```python
from build123d import *

# Parameters (mm, degrees)
SKETCH5_W           = 90
SKETCH5_H           = 80
BOSS_EXTRUDE4_DEPTH = 13
BOSS_EXTRUDE5_DEPTH = 80
CHAMFER1_SIZE       = 7
SKETCH13_R          = 2
CUT_EXTRUDE4_DEPTH  = 20
SKETCH14_R          = 2
CUT_EXTRUDE8_DEPTH  = 20


with BuildPart() as part:
    # Sketch5 → Boss-Extrude4 (new body)
    with BuildSketch(Plane.XY):
        with Locations((0, -5.742449829)):
            Rectangle(SKETCH5_W, SKETCH5_H)
    extrude(amount=BOSS_EXTRUDE4_DEPTH)

    # Sketch6 → Boss-Extrude5 (add, through all)
    with BuildSketch(Plane.XZ.offset(45.742449829)):
        Polygon((-45, 13), (-38, 20), (38, 20), (45, 13), (45, 0), (-45, 0), align=None)
    extrude(amount=-BOSS_EXTRUDE5_DEPTH)

    # Chamfer1
    chamfer1_edges = [part.edges().sort_by_distance(p)[0] for p in [
        (0, -45.742449829, 20),
        (0, 34.257550171, 20),
    ]]
    chamfer(chamfer1_edges, length=CHAMFER1_SIZE)

    # Sketch13 → Cut-Extrude4 (cut)
    with BuildSketch(Plane(origin=(0, 0, 0), x_dir=(-1, 0, 0), z_dir=(0, 0, -1))):
        with Locations((0, -32.742449829)):
            Circle(SKETCH13_R)
    extrude(amount=-CUT_EXTRUDE4_DEPTH, mode=Mode.SUBTRACT)

    # Sketch14 → Cut-Extrude8 (cut)
    with BuildSketch(Plane(origin=(0, 0, 0), x_dir=(-1, 0, 0), z_dir=(0, 0, -1))):
        with Locations((-33, 18.257550171)):
            Circle(SKETCH14_R)
        with Locations((33, 18.257550171)):
            Circle(SKETCH14_R)
    extrude(amount=-CUT_EXTRUDE8_DEPTH, mode=Mode.SUBTRACT)


solid = part.part
```
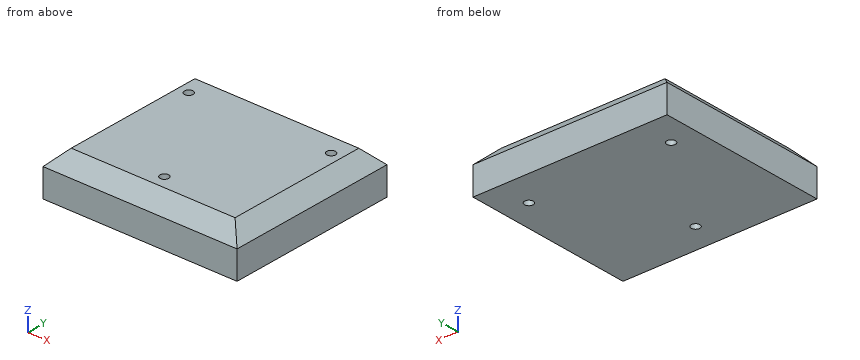
Design review of the part built by this model. Coordinates are the model's own, in mm. Round coordinates to 2 decimals unless told otherwise and drop trailing zeros. Write each loop counter-clockwise with the first axis right and the second up, starting at its lowest first coordinate (ties: lowest second). Pieces come first, ordered by that corner, then holes.
Item 1: We need section B-B on z = 16.5. Write out the cut boundary in (x, y), and give its area (3 significant figures).
Item 2: We need section C-C on x = -26.5. Write out the cut boundary in (y, z).
Item 3: For probe 1 along Y at (x, z) = (33, 5); probe 2 along Y at (x, z) = (0, 9.5); probe 3 along X at (y, z) = (19, 3), list the stretches that pass through material, from the lowest coordinate up.
Item 4: Clearance check with a flat-ended pin moving along its axis: pin 1 Ø10 at (x, y) = (0.5, 11.5) entering from -Z. State where the tip first meets the part, or that it passes through.
Item 5: We need section A-A on x = 0. Write out the cut boundary in (y, z), and give its area (3 significant figures).
Item 6: We need section D-D on y = -13. Write out the cut boundary in (x, z).
Returned:
1. outline: (-41.5, -42.24) - (41.5, -42.24) - (41.5, 30.76) - (-41.5, 30.76) - close; hole circle Ø4 at (-33, 18.26); hole circle Ø4 at (0, -32.74); hole circle Ø4 at (33, 18.26)
1. area: 6,020 mm2
2. outline: (-45.74, 0) - (34.26, 0) - (34.26, 13) - (27.26, 20) - (-38.74, 20) - (-45.74, 13) - close
3. probe 1: y = -45.74 to 16.26, 20.26 to 34.26
3. probe 2: y = -45.74 to -34.74, -30.74 to 34.26
3. probe 3: x = -45 to -34.86, -31.14 to 31.14, 34.86 to 45
4. pin 1: stops at z = 0
5. outline: (-45.74, 0) - (-34.74, 0) - (-34.74, 20) - (-38.74, 20) - (-45.74, 13) - close; (-30.74, 0) - (34.26, 0) - (34.26, 13) - (27.26, 20) - (-30.74, 20) - close
5. area: 1,470 mm2
6. outline: (-45, 0) - (45, 0) - (45, 13) - (38, 20) - (-38, 20) - (-45, 13) - close
